```python
from build123d import *

# Parameters (mm, degrees)
MAIN_DEPTH             = 5
MAKERBEAMFIX_DEPTH     = 20
SKETCH2_R              = 1.5
MAKERBEAMFIXHOLE_DEPTH = 30
FILLET1_R              = 2


with BuildPart() as part:
    # Esquisse1 → Main (new body, symmetric)
    with BuildSketch(Plane.XY):
        Polygon((3, 0), (3, 5), (15, 5), (15, 0), (22, 0), (22, 5), (34, 5), (34, 0), (41, 0), (41, 5), (53, 5), (53, 0), (60, 0), (60, 5), (72, 5), (72, 8), (0, 8), (0, 0), align=None)
    extrude(amount=MAIN_DEPTH, both=True)

    # Sketch1 → MakerBeamFix (add, symmetric)
    with BuildSketch(Plane.XY):
        Polygon((67, 14), (72, 14), (72, 10.45), (73, 10.45), (73, 7.55), (72, 7.55), (72, 5), (67, 5), align=None)
    extrude(amount=MAKERBEAMFIX_DEPTH, both=True)

    # Sketch2 → MakerBeamFixHole (cut)
    with BuildSketch(Plane(origin=(73, 0, 0), x_dir=(0, 0, -1), z_dir=(1, 0, 0))):
        with Locations((-17, 9)):
            Circle(SKETCH2_R)
        with Locations((17, 9)):
            Circle(SKETCH2_R)
    extrude(amount=-MAKERBEAMFIXHOLE_DEPTH, mode=Mode.SUBTRACT)

    # Fillet1
    fillet1_edges = [part.edges().sort_by_distance(p)[0] for p in [
        (67, 6.5, -5),
        (67, 6.5, 5),
        (67, 8, 0),
    ]]
    fillet(fillet1_edges, radius=FILLET1_R)


solid = part.part
```
Could you check a few things on this model? Use its own coordinates, in mm. A direction names the side the tool comes from. Give positions to 0.01 mm unless a question says otherwise; leave off trailing zeros. Loops run counter-clockwise (first coordinate to the right, second up) from the corner with the lowest first, then second, coordinate; pieces in that order, holes last. Notation, with made-up numbers: (62, 45) - (69, 45) arc R8 ccw to (69, 58) - close; hole circle Ø7 at (-10, 43). An arc over 180 degrees is marked (long way). Use one line per item in the form item = value.
1. I'm going to push flat-ended pins straight in: pin 1 Ø1.5 at (y, z) = (2, 0.5) entering from +X; pin 2 Ø3 at (x, y) = (26, 3) entering from +Z; pin 3 Ø1 at (y, z) = (8, -8.5) entering from -X; pin 4 Ø1.1 at (x, z) = (72.5, -18.5) entering from -Y. Where does each tip first touch, or does it pass through?
Response values:
pin_1 = 60
pin_2 = through
pin_3 = 67
pin_4 = 5
2. I need wall thicknesses on probe 1 along X at (y, z) = (1.75, -4.5); probe 2 along Y at (x, z) = (70, -17); probe 3 along X at (y, z) = (6.5, 15). Which ranges of each line are inside material? Lowest first, please.
Response values:
probe_1 = 0 to 3, 15 to 22, 34 to 41, 53 to 60
probe_2 = 5 to 7.5, 10.5 to 14
probe_3 = 67 to 72
3. I want a section at C-C (x = 39). Please give me the cut outline in (y, z), and give its area (3 significant figures).
Response values:
outline = (0, -5) - (8, -5) - (8, 5) - (0, 5) - close
area = 80.0 mm²
4. I want a section at A-A (z = 14). Please give me the cut outline in (x, y), and give its area (3 significant figures).
Response values:
outline = (67, 5) - (72, 5) - (72, 7.55) - (73, 7.55) - (73, 10.45) - (72, 10.45) - (72, 14) - (67, 14) - close
area = 47.9 mm²
5. I want a section at D-D (z = -2). Please give me the cut outline in (x, y).
Response values:
outline = (0, 0) - (3, 0) - (3, 5) - (15, 5) - (15, 0) - (22, 0) - (22, 5) - (34, 5) - (34, 0) - (41, 0) - (41, 5) - (53, 5) - (53, 0) - (60, 0) - (60, 5) - (72, 5) - (72, 7.55) - (73, 7.55) - (73, 10.45) - (72, 10.45) - (72, 14) - (67, 14) - (67, 10) arc R2 cw to (65, 8) - (0, 8) - close
6. On a 3-axis mill with a long thin cutter (end or side, diameter ignored), from which of +Z, -Z, +X, -X, +Y, -Y can I reach the whole of each face in a straight line? I mean faces 5 (the face through (41, 2, 0)), 6 (the face through (32, 6, -5)), 7 (the face through (33, 8, 0)), 8 (the face through (60, 2, 0)). Say none if no direction works.
Response values:
face_5 = +Z, -Z, -Y
face_6 = -Z, -X, +Y, -Y
face_7 = +Z, -Z, -X, +Y
face_8 = +Z, -Z, +X, -Y
7. I want a section at B-B (y = 9). Please give me the cut outline in (x, z).
Response values:
outline = (66.73, -6) arc R2 cw to (67, -7) - (67, -15.5) - (73, -15.5) - (73, 15.5) - (67, 15.5) - (67, 7) arc R2 cw to (66.73, 6) - close; (67, -20) - (73, -20) - (73, -18.5) - (67, -18.5) - close; (67, 18.5) - (73, 18.5) - (73, 20) - (67, 20) - close
8. Thinking about a two-plate mould opening in X: for faces 1 (the face through (3, 2, 0)), 2 (the face through (73, 9, 19)), 3 (the face through (66.43, 8.6, -0.1)), 4 (the face through (69, 14, 0)), which applies, released by +X, released by -X, zero draft, split by the parting line, or undercut?
Response values:
face_1 = undercut
face_2 = released by +X
face_3 = released by -X
face_4 = zero draft
